Input: part model. Units: mm. Frame: model coordinates. Face numbers are marked on the shaded views. A direction names the side the tool comes from. Round coordinates to 2 decimals unless told otherwise and drop trailing zeros. Loops run counter-clockwise (first coordinate to the right, second up) from the corner with the lowest first, then second, coordinate; pieces in that order, holes last. Notation, with made-up numbers: M 63,36.25 L 116,36.25 A15 cw 116,47.25 Z; hole C 9,66 d2. An arc over 180 degrees is marked long. Put each result on its own line as item: value. Start each with the question number.
1) Section C-C on z = -7.5. Output: boundary loops of the cut face in (x, y), plus the area to 3 significant figures.
2) Section A-A on y = 18. Output: boundary loops of the cut face in (x, z), plus the area to 3 significant figures.
3) Pin query (flat end, axial travel): pin 1 (2.5 mm diameter, centred on x = 5.5, z = 7, fed in from -Y); pin 2 (4 mm diameter, centred on x = 4, y = 12.5, fed in from +Z); pin 3 (12.5 mm diameter, centred on y = 18, z = 0.5, fed in from +X); pin 4 (5.5 mm diameter, centred on x = 12, y = 47.5, fed in from +Z). Return the tip coordinate at first contact, or that it passes through.
4) Line query: probe 1 along Y at (x, z) = (5, -7.5); probe 2 along Y at (x, z) = (12, 5.4); probe 3 along X at (y, z) = (45, 4.1). Output: solid intervals per line, ascending.
5) Section D-D on x = 13.5. Output: boundary loops of the cut face in (y, z).
6) Reachability of the marked faces 1, 2, 3, 4 and 5 from +Z, -Z, +X, -X, +Y, -Y: full face, straight path, thin tool, end or side. Return the list, or none.
7) Section B-B on x = 7.25. Output: boundary loops of the cut face in (y, z), plus the area to 3 significant figures.
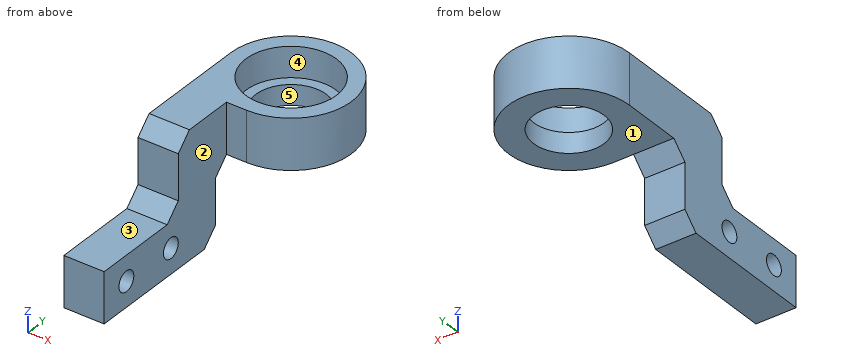
from build123d import *

# Parameters (mm, degrees)
SKETCH_1_R               = 7
EXTRUDE_1_DEPTH          = 12.5
CUT_EXTRUDE_3_DEPTH      = 64.097147321
CUT_EXTRUDE_3_DEPTH_BACK = 64.097147321
SKETCH_5_OUTSIDE_W       = 40.342
SKETCH_5_OUTSIDE_H       = 72.342
SKETCH_2_R               = 2
CUT_EXTRUDE_1_DEPTH      = 64.097147321
SKETCH_4_R               = 9
CUT_EXTRUDE_2_DEPTH      = 6
CHAMFER_1_SIZE           = 3


with BuildPart() as part:
    # 草图1 → 凸台-拉伸1 (new, symmetric)
    with BuildSketch(Plane.XY):
        with BuildLine():
            Line((0, 0), (8, 0))
            Line((8, 0), (8, 33))
            Line((8, 33), (12, 33))
            ThreePointArc((12, 33), (20.485281374, 53.485281374), (0, 45))
            Line((0, 45), (0, 0))
        make_face()
        with Locations((12, 45)):
            Circle(SKETCH_1_R, mode=Mode.SUBTRACT)
    extrude(amount=EXTRUDE_1_DEPTH, both=True)

    # 草图5 outside → 切除-拉伸3 (cut, two sides: drawn at the far end of the back side and taken through both)
    with BuildSketch(Plane(origin=(0, 0, 0), x_dir=(0, 0, -1), z_dir=(1, 0, 0)).offset(-CUT_EXTRUDE_3_DEPTH_BACK)):
        with Locations((0, 28.5)):
            Rectangle(SKETCH_5_OUTSIDE_W, SKETCH_5_OUTSIDE_H)
        Polygon((-12.5, 57), (-2.5, 57), (-2.5, 30), (12.5, 30), (12.5, 0), (2.5, 0), (2.5, 20), (-12.5, 20), align=None, mode=Mode.SUBTRACT)
    extrude(amount=CUT_EXTRUDE_3_DEPTH + CUT_EXTRUDE_3_DEPTH_BACK, mode=Mode.SUBTRACT)

    # 草图2 → 切除-拉伸1 (cut, through all)
    with BuildSketch(Plane.ZY):
        with Locations((-7.5, 18)):
            Circle(SKETCH_2_R)
        with Locations((-7.5, 6)):
            Circle(SKETCH_2_R)
    extrude(amount=-CUT_EXTRUDE_1_DEPTH, mode=Mode.SUBTRACT)

    # 草图4 → 切除-拉伸2 (cut)
    with BuildSketch(Plane.XY.offset(12.5)):
        with Locations((12, 45)):
            Circle(SKETCH_4_R)
    extrude(amount=-CUT_EXTRUDE_2_DEPTH, mode=Mode.SUBTRACT)

    # 倒角1
    chamfer_1_edges = [part.edges().sort_by_distance(p)[0] for p in [
        (4, 30, 2.5),
        (4, 30, -12.5),
        (4, 20, -2.5),
        (4, 20, 12.5),
    ]]
    chamfer(chamfer_1_edges, length=CHAMFER_1_SIZE)


solid = part.part
Geometry results:
1. outline: M 0,0 L 8,0 L 8,4 L 0,4 Z; M 0,8 L 8,8 L 8,16 L 0,16 Z; M 0,20 L 8,20 L 8,30 L 0,30 Z
1. area: 176 mm²
2. outline: M 0,-12.5 L 8,-12.5 L 8,-9.5 L 0,-9.5 Z; M 0,-5.5 L 8,-5.5 L 8,-1.5 L 0,-1.5 Z
2. area: 56.0 mm²
3. pin 1: stops at y = 20
3. pin 2: stops at z = -2.5
3. pin 3: stops at x = 8
3. pin 4: passes through
4. probe 1: y = 0 to 4, 8 to 16, 20 to 30
4. probe 2: y = 33 to 38, 52 to 57
4. probe 3: x = 0 to 5, 19 to 24
5. outline: M 33.09,2.5 L 38.16,2.5 L 38.16,6.5 L 36.13,6.5 L 36.13,12.5 L 33.09,12.5 Z; M 51.84,2.5 L 56.91,2.5 L 56.91,12.5 L 53.87,12.5 L 53.87,6.5 L 51.84,6.5 Z
6. face 1: -Z, +X, -X, +Y
6. face 2: +Z, -Z, +X, -Y
6. face 3: +Z, +X, -X, -Y
6. face 4: +Z
6. face 5: +Z, -Z
7. outline: M 0,-12.5 L 27,-12.5 L 30,-9.5 L 30,-0.5 L 33,2.5 L 39.86,2.5 L 39.86,6.5 L 37.36,6.5 L 37.36,12.5 L 23,12.5 L 20,9.5 L 20,0.5 L 17,-2.5 L 0,-2.5 Z; M 50.14,2.5 L 56.02,2.5 L 56.02,12.5 L 52.64,12.5 L 52.64,6.5 L 50.14,6.5 Z; hole C 6,-7.5 d4; hole C 18,-7.5 d4
7. area: 552 mm²
